from build123d import *

# Parameters (mm, degrees)
SKETCH2_W           = 5
SKETCH2_H           = 13.5
BOSS_EXTRUDE3_DEPTH = 1
SKETCH2_7_W         = 26
SKETCH2_7_H         = 13.5
BOSS_EXTRUDE6_DEPTH = 4.951
CUT_EXTRUDE2_START  = 4.951
CUT_EXTRUDE2_DEPTH  = 1.951
CUT_EXTRUDE3_START  = 3
CUT_EXTRUDE3_DEPTH  = 0.5
M2_TAPPED_HOLE1_D   = 1.6
BOX_OUTLINE_R       = 0.8
BOX_DEPTH           = 3
BOX_2_OUTLINE_W     = 5
BOX_2_OUTLINE_H     = 13.5
BOX_2_OUTLINE_H_2   = 27
BOX_2_DEPTH         = 1
BOX_START           = 3
BOX_3_DEPTH         = 1.951
BOX_START_2         = 1
BOX_4_DEPTH         = 1.5


# Read off the part's stored shape, not the designer's step: box
with BuildPart() as part:
    # Sketch2 → Boss-Extrude3 (new body)
    with BuildSketch(Plane(origin=(0, 0, 0), x_dir=(1, 0, 0), z_dir=(0, 1, 0))):
        with Locations((28.5, 6.75)):
            Rectangle(SKETCH2_W, SKETCH2_H)
    extrude(amount=BOSS_EXTRUDE3_DEPTH)

    # Sketch2<7> → Boss-Extrude6 (add)
    with BuildSketch(Plane(origin=(0, 0, 0), x_dir=(1, 0, 0), z_dir=(0, 1, 0))):
        with Locations((13, 6.75)):
            Rectangle(SKETCH2_7_W, SKETCH2_7_H)
    extrude(amount=BOSS_EXTRUDE6_DEPTH)

    # Sketch2<9> → Cut-Extrude2 (cut)
    with BuildSketch(Plane(origin=(0, 0, 0), x_dir=(1, 0, 0), z_dir=(0, 1, 0)).offset(CUT_EXTRUDE2_START)):
        Polygon((3.15, 0), (25, 0), (25, 12.5), (0, 12.5), (0, 3.15), (2.35, 3.15), (3.15, 2.35), align=None)
        Polygon((0, 0), (3.15, 0), (3.15, 2.35), (2.35, 3.15), (0, 3.15), align=None)
    extrude(amount=-CUT_EXTRUDE2_DEPTH, mode=Mode.SUBTRACT)

    # Sketch2<12> → Cut-Extrude3 (cut)
    with BuildSketch(Plane(origin=(0, 0, 0), x_dir=(1, 0, 0), z_dir=(0, 1, 0)).offset(CUT_EXTRUDE3_START)):
        Polygon((0, 0), (3.15, 0), (3.15, 2.35), (2.35, 3.15), (0, 3.15), align=None)
    extrude(amount=-CUT_EXTRUDE3_DEPTH, mode=Mode.SUBTRACT)

    # M2 Tapped Hole1 (through all)
    with Locations(Plane(origin=(0, 3, 0), x_dir=(1, 0, 0), z_dir=(0, 1, 0))):
        with Locations((21.5, 9)):
            Hole(M2_TAPPED_HOLE1_D / 2)

    # box outline → box (add)
    with BuildSketch(Plane(origin=(0, 0, 0), x_dir=(1, 0, 0), z_dir=(0, 1, 0))):
        Polygon((-26, -13.5), (26, -13.5), (26, 0), (3.15, 0), (3.15, -2.35), (2.35, -3.15), (-2.35, -3.15), (-3.15, -2.35), (-3.15, 2.35), (-2.35, 3.15), (0, 3.15), (0, 13.5), (-26, 13.5), align=None)
        with Locations((-21.5, -9)):
            Circle(BOX_OUTLINE_R, mode=Mode.SUBTRACT)
        with Locations((21.5, -9)):
            Circle(BOX_OUTLINE_R, mode=Mode.SUBTRACT)
        with Locations((-21.5, 9)):
            Circle(BOX_OUTLINE_R, mode=Mode.SUBTRACT)
    extrude(amount=BOX_DEPTH)

    # box 2 outline → box 2 (add)
    with BuildSketch(Plane(origin=(0, 0, 0), x_dir=(1, 0, 0), z_dir=(0, 1, 0))):
        with Locations((28.5, -6.75)):
            Rectangle(BOX_2_OUTLINE_W, BOX_2_OUTLINE_H)
        with Locations((-28.5, 0)):
            Rectangle(BOX_2_OUTLINE_W, BOX_2_OUTLINE_H_2)
        Polygon((3.15, -2.35), (3.15, 0), (0, 0), (0, 3.15), (-2.35, 3.15), (-3.15, 2.35), (-3.15, -2.35), (-2.35, -3.15), (2.35, -3.15), align=None)
    extrude(amount=BOX_2_DEPTH)

    # box 3 outline → box 3 (add)
    with BuildSketch(Plane(origin=(0, 0, 0), x_dir=(1, 0, 0), z_dir=(0, 1, 0)).offset(BOX_START)):
        Polygon((-26, -13.5), (26, -13.5), (26, 0), (25, 0), (25, -12.5), (-25, -12.5), (-25, 12.5), (0, 12.5), (0, 13.5), (-26, 13.5), align=None)
    extrude(amount=BOX_3_DEPTH)

    # box 4 outline → box 4 (add)
    with BuildSketch(Plane(origin=(0, 0, 0), x_dir=(1, 0, 0), z_dir=(0, 1, 0)).offset(BOX_START_2)):
        Polygon((3.15, -2.35), (3.15, 0), (0, 0), (0, 3.15), (-2.35, 3.15), (-3.15, 2.35), (-3.15, -2.35), (-2.35, -3.15), (2.35, -3.15), align=None)
    extrude(amount=BOX_4_DEPTH)


solid = part.part
Verification items for the finished model (mm, model axes). A direction names the side the tool comes from. Coordinates: 2 decimals unless noted, no trailing zeros. Loops run counter-clockwise (first coordinate to the right, second up) from the corner with the lowest first, then second, coordinate; pieces in that order, holes last. Notation, with made-up numbers: (43.5, -13.5) -> (76.5, -13.5) arc R24 cw to (76.5, -2.5) -> close; hole circle Ø11 at (-10.75, 37). An arc over 180 degrees is marked (long way). Write each question's results on one line, items separated by ' | '.
Item 1: Material ranges on L1, parallel to X at y = 2.15, z = 9; L2, parallel to Z at x = -21.5, y = 1.6; L3, parallel to X at y = 0.7, z = -9, recorded low to high.
Found:
L1: x = -26 to -22.3, -20.7 to 20.7, 22.3 to 26 | L2: z = -13.5 to -9.8, -8.2 to 8.2, 9.8 to 13.5 | L3: x = -31 to -22.3, -20.7 to 20.7, 22.3 to 31
Item 2: Tool access check on faces 1 (the face through (28, 1, 0)), 2 (the face through (-6, 3, 0)), 3 (the face through (-26, 3, 0)). Record the directions out of +Z, -Z, +X, -X, +Y, -Y that give a thin tool (end or side, any length) a straight path to the whole face; none if there is none.
Found:
face 1: +Z, -Z, +X, +Y | face 2: +Y | face 3: +Z, -Z, -X, +Y
Item 3: Section check A-A, the plane z = 9. Enter the section's corners in (x, y), plus the area to 3 significant figures.
Found:
outline: (-31, 0) -> (-22.3, 0) -> (-22.3, 3) -> (-25, 3) -> (-25, 4.95) -> (-26, 4.95) -> (-26, 1) -> (-31, 1) -> close; (-20.7, 0) -> (20.7, 0) -> (20.7, 3) -> (-20.7, 3) -> close; (22.3, 0) -> (31, 0) -> (31, 1) -> (26, 1) -> (26, 4.95) -> (25, 4.95) -> (25, 3) -> (22.3, 3) -> close | area: 160 mm2
Item 4: Gauge pin test, flat ends, axial feed: pin 1 (2 mm diameter, centred on y = 4.5, z = 7.5, fed in from -X); pin 2 (2.5 mm diameter, centred on x = -28.5, z = 2.5, fed in from +Y); pin 3 (1.4 mm diameter, centred on x = -21.5, z = -9, fed in from -Y); pin 4 (5 mm diameter, centred on x = -1, z = 1.5, fed in from +Y). Record the tip position at first contact, or that the pin passes through.
Found:
pin 1: stops at x = -26 | pin 2: stops at y = 1 | pin 3: passes through | pin 4: stops at y = 3
Item 5: Section check B-B, the plane x = 21.5. Enter the section's corners in (y, z), plus the area to 3 significant figures.
Found:
outline: (0, -13.5) -> (4.95, -13.5) -> (4.95, -12.5) -> (3, -12.5) -> (3, -9.8) -> (0, -9.8) -> close; (0, -8.2) -> (3, -8.2) -> (3, 8.2) -> (0, 8.2) -> close; (0, 9.8) -> (3, 9.8) -> (3, 12.5) -> (4.95, 12.5) -> (4.95, 13.5) -> (0, 13.5) -> close | area: 75.3 mm2
Item 6: Mould release check, pull along Z, two halves, no side actions. Record for faces 4 (the face through (21.396, 1.479, 8.207)), 5 (the face through (26, 3, 0)), 6 (the face through (0, 2, 13.5)), 7 (the face through (25, 4, 0)): +Z half, -Z half, draft (parallel to the pull), parting line (faces both ways), or undercut.
Found:
face 4: undercut | face 5: draft | face 6: +Z half | face 7: undercut
Item 7: Section check D-D, the plane z = -11.5. Enter the section's corners in (x, y), plus the area to 3 significant figures.
Found:
outline: (-31, 0) -> (31, 0) -> (31, 1) -> (26, 1) -> (26, 4.95) -> (25, 4.95) -> (25, 3) -> (-25, 3) -> (-25, 4.95) -> (-26, 4.95) -> (-26, 1) -> (-31, 1) -> close | area: 170 mm2
Item 8: Section check C-C, the plane y = 1.65. Enter the section's corners in (x, z), plus the area to 3 significant figures.
Found:
outline: (-26, -13.5) -> (26, -13.5) -> (26, 13.5) -> (-26, 13.5) -> close; hole circle Ø1.6 at (-21.5, -9); hole circle Ø1.6 at (-21.5, 9); hole circle Ø1.6 at (21.5, -9); hole circle Ø1.6 at (21.5, 9) | area: 1,400 mm2
